Part model, mm, in its own coordinate system. A direction names the side the tool comes from. Round coordinates to 2 decimals unless told otherwise and drop trailing zeros. Loops run counter-clockwise (first coordinate to the right, second up) from the corner with the lowest first, then second, coordinate; pieces in that order, holes last. Notation, with made-up numbers: (-2, 28) - (10, 28) arc R31 ccw to (10, 59) - close; hole circle Ø9 at (8, 44). An arc over 180 degrees is marked (long way). Put each result on its own line as item: value.
from build123d import *

# Parameters (mm, degrees)
RESSALTO_EXTRUS_O1_DEPTH                     = 200
CORTE_EXTRUS_O3_REACH                        = 224.463
ESBO_O4_R                                    = 1.825
CORTE_EXTRUS_O5_REACH                        = 224.463
ESBO_O6_R                                    = 6.0125
BROCA_DE_ROSQUEAR_PARA_TARRAXA_DE_M3X0_5_D   = 2.5
ESBO_O15_W                                   = 12
ESBO_O15_H                                   = 2.152025528
CORTE_EXTRUS_O7_DEPTH                        = 16.7
CORTE_EXTRUS_O8_REACH                        = 224.463
ESBO_O5_R                                    = 6.0125
BROCA_DE_ROSQUEAR_PARA_TARRAXA_DE_M3_2_D     = 2.5
BROCA_DE_ROSQUEAR_PARA_TARRAXA_DE_M3_2_DEPTH = 2
BROCA_DE_ROSQUEAR_PARA_TARRAXA_DE_M3_3_D     = 2.5
BROCA_DE_ROSQUEAR_PARA_TARRAXA_DE_M3_3_DEPTH = 2
BROCA_DE_ROSQUEAR_PARA_TARRAXA_DE_M3_4_D     = 2.5
BROCA_DE_ROSQUEAR_PARA_TARRAXA_DE_M3_4_DEPTH = 2
BROCA_DE_ROSQUEAR_PARA_TARRAXA_DE_M3_5_D     = 2.5
BROCA_DE_ROSQUEAR_PARA_TARRAXA_DE_M3_5_DEPTH = 2


with BuildPart() as part:
    # Esboço1 → Ressalto-extrusão1 (new body)
    with BuildSketch(Plane.XY):
        Polygon((-54.740307174, -0.6), (-54.740307174, 63.2), (-71.440307174, 63.2), (-71.440307174, 65.2), (-54.740307174, 65.2), (-54.740307174, 71.2), (-71.440307174, 71.2), (-71.440307174, 73.2), (-54.740307174, 73.2), (-54.740307174, 79.2), (-73.740307174, 79.2), (-73.740307174, 83), (-71.740307174, 83), (-71.740307174, 81.2), (-59.940307174, 81.2), (-59.940307174, 91.6), (-71.740307174, 91.6), (-71.740307174, 89.8), (-73.740307174, 89.8), (-73.740307174, 93.6), (-54.940307174, 93.6), (-54.940307174, 91.6), (-56.940307174, 91.6), (-56.940307174, 83.4), (-44.540307174, 83.4), (-44.540307174, 91.6), (-46.540307174, 91.6), (-46.540307174, 93.6), (-27.740307174, 93.6), (-27.740307174, 89.8), (-29.740307174, 89.8), (-29.740307174, 91.6), (-41.540307174, 91.6), (-41.540307174, 81.2), (-29.740307174, 81.2), (-29.740307174, 83), (-27.740307174, 83), (-27.740307174, 79.2), (-46.740307174, 79.2), (-46.740307174, 71.9), (-30.040307174, 71.9), (-30.040307174, 69.9), (-46.740307174, 69.9), (-46.740307174, 62.6), (-30.040307174, 62.6), (-30.040307174, 60.6), (-46.740307174, 60.6), (-46.740307174, 53.3), (-30.040307174, 53.3), (-30.040307174, 51.3), (-46.740307174, 51.3), (-46.740307174, 11.3), (-30.040307174, 11.3), (-30.040307174, 9.3), (-46.740307174, 9.3), (-46.740307174, 2), (-30.040307174, 2), (-30.040307174, 0), (-46.740307174, 0), (-46.740307174, -7.3), (-30.040307174, -7.3), (-30.040307174, -9.3), (-46.740307174, -9.3), (-46.740307174, -16.6), (-27.740307174, -16.6), (-27.740307174, -20.4), (-29.740307174, -20.4), (-29.740307174, -18.6), (-41.540307174, -18.6), (-41.540307174, -29), (-29.740307174, -29), (-29.740307174, -27.2), (-27.740307174, -27.2), (-27.740307174, -31), (-46.540307174, -31), (-46.540307174, -29), (-44.540307174, -29), (-44.540307174, -20.8), (-56.940307174, -20.8), (-56.940307174, -29), (-54.940307174, -29), (-54.940307174, -31), (-73.740307174, -31), (-73.740307174, -27.2), (-71.740307174, -27.2), (-71.740307174, -29), (-59.940307174, -29), (-59.940307174, -18.6), (-71.740307174, -18.6), (-71.740307174, -20.4), (-73.740307174, -20.4), (-73.740307174, -16.6), (-54.740307174, -16.6), (-54.740307174, -10.6), (-71.440307174, -10.6), (-71.440307174, -8.6), (-54.740307174, -8.6), (-54.740307174, -2.6), (-71.440307174, -2.6), (-71.440307174, -0.6), align=None)
    extrude(amount=RESSALTO_EXTRUS_O1_DEPTH)

    # Esboço4 → Corte-extrusão3 (cut, up to next)
    with BuildSketch(Plane.ZY.offset(54.740307174), mode=Mode.PRIVATE) as corte_extrus_o3_sk1:
        with Locations(Location((104, 50.1, 0), (0, 0, 270))):
            Circle(ESBO_O4_R)
    corte_extrus_o3_tool1 = extrude(corte_extrus_o3_sk1.sketch, amount=-CORTE_EXTRUS_O3_REACH, mode=Mode.PRIVATE) & part.part
    add(corte_extrus_o3_tool1.solids().sort_by_distance((-54.740307, 50.1, 104))[0], mode=Mode.SUBTRACT)

    # Esboço6 → Corte-extrusão5 (cut, up to next)
    with BuildSketch(Plane.ZY.offset(54.740307174), mode=Mode.PRIVATE) as corte_extrus_o5_sk1:
        with Locations(Location((104, 12.5, 0), (0, 0, 270))):
            Circle(ESBO_O6_R)
    corte_extrus_o5_tool1 = extrude(corte_extrus_o5_sk1.sketch, amount=-CORTE_EXTRUS_O5_REACH, mode=Mode.PRIVATE) & part.part
    add(corte_extrus_o5_tool1.solids().sort_by_distance((-54.740307, 12.5, 104))[0], mode=Mode.SUBTRACT)

    # Broca de rosquear para tarraxa de M3x0.5 (through all)
    with Locations(Plane.ZY.offset(54.740307174)):
        with Locations((6, 5.9), (6, 58.2)):
            Hole(BROCA_DE_ROSQUEAR_PARA_TARRAXA_DE_M3X0_5_D / 2)

    # Esboço15 → Corte-extrusão7 (cut)
    with BuildSketch(Plane(origin=(-30.040307174, 0, 0), x_dir=(0, 0, -1), z_dir=(1, 0, 0))):
        with Locations((-104.566575702, 52.223987236)):
            Rectangle(ESBO_O15_W, ESBO_O15_H)
    extrude(amount=-CORTE_EXTRUS_O7_DEPTH, mode=Mode.SUBTRACT)

    # Esboço5 → Corte-extrusão8 (cut, up to next)
    with BuildSketch(Plane.ZY.offset(54.740307174), mode=Mode.PRIVATE) as corte_extrus_o8_sk1:
        with Locations(Location((130, 50.1, 0), (0, 0, 270))):
            Circle(ESBO_O5_R)
    corte_extrus_o8_tool1 = extrude(corte_extrus_o8_sk1.sketch, amount=-CORTE_EXTRUS_O8_REACH, mode=Mode.PRIVATE) & part.part
    add(corte_extrus_o8_tool1.solids().sort_by_distance((-54.740307, 50.1, 130))[0], mode=Mode.SUBTRACT)

    # Broca de rosquear para tarraxa de M3 2
    with Locations(Plane.XZ.offset(31)):
        with Locations((-64.286083069, 189.76), (-37.140307173, 189.76)):
            Hole(BROCA_DE_ROSQUEAR_PARA_TARRAXA_DE_M3_2_D / 2, depth=BROCA_DE_ROSQUEAR_PARA_TARRAXA_DE_M3_2_DEPTH)

    # Broca de rosquear para tarraxa de M3 3
    with Locations(Plane(origin=(0, 93.6, 0), x_dir=(-1, 0, 0), z_dir=(0, 1, 0))):
        with Locations((37.140307173, 189.76), (64.340307173, 189.76)):
            Hole(BROCA_DE_ROSQUEAR_PARA_TARRAXA_DE_M3_3_D / 2, depth=BROCA_DE_ROSQUEAR_PARA_TARRAXA_DE_M3_3_DEPTH)

    # Broca de rosquear para tarraxa de M3 4
    with Locations(Plane.XZ.offset(31)):
        with Locations((-64.340307174, 18.36), (-64.340307174, 6.36)):
            Hole(BROCA_DE_ROSQUEAR_PARA_TARRAXA_DE_M3_4_D / 2, depth=BROCA_DE_ROSQUEAR_PARA_TARRAXA_DE_M3_4_DEPTH)

    # Broca de rosquear para tarraxa de M3 5
    with Locations(Plane(origin=(0, 93.6, 0), x_dir=(-1, 0, 0), z_dir=(0, 1, 0))):
        with Locations((64.340307174, 18.36), (64.340307174, 6.36)):
            Hole(BROCA_DE_ROSQUEAR_PARA_TARRAXA_DE_M3_5_D / 2, depth=BROCA_DE_ROSQUEAR_PARA_TARRAXA_DE_M3_5_DEPTH)


solid = part.part
1. Two-plate mould, pull along Z, no slides. Class faces 1 (the flat face through (-36, 81.2, 99)), 2 (the cylindrical face through (-48.05, 51.4, 124.13)), 3 (the flat face through (-54, 32, 0)): pulls with the +Z half, pulls with the -Z half, needs draft (parallel to the pull), parting line crosses it, or undercut.
A:
face 1: needs draft
face 2: undercut
face 3: pulls with the -Z half
2. Band-saw the part on B-B (y = 33.5). List the corners of the cut face in (x, z).
A:
outline: (-54.74, 0) - (-46.74, 0) - (-46.74, 200) - (-54.74, 200) - close
3. Pin check, flat tips, straight feed: P1, Ø4, axis at y = 27.5, z = 41, coming from the +X side; P2, Ø3, axis at x = -49.5, z = 73, coming from the +Y side; P3, Ø1.6, axis at y = 52.5, z = 116.5, coming from the +X side. Stop position of each tip, or through.
A:
P1: stops at x = -46.74
P2: stops at y = 83.4
P3: stops at x = -30.04
4. Probe line 1 along Z through (x, y) = (-50.75, 50.1) (1 decimal); line 2 along X through (y, z) = (84.5, 96.5); line 3 along X through (y, z) = (-30.25, 189.76). List the from-to ranges inside material, lowest first. Write a range as [from, to].
A:
line 1: z = [0, 102.2], [105.8, 124], [136, 200]
line 2: x = [-59.94, -56.94], [-44.54, -41.54]
line 3: x = [-73.74, -65.54], [-63.04, -54.94], [-46.54, -38.39], [-35.89, -27.74]
5. Tool access for faces 4 (the flat face through (-38, 60.6, 99)), 5 (the flat face through (-63, -8.6, 99)), 6 (the flat face through (-66, -29, 99)), 7 (the flat face through (-73.74, 92, 99)): list every direction of +Z, -Z, +X, -X, +Y, -Y with a clear straight run to the whole face (end or side of a thin tool).
A:
face 4: +Z, -Z, +X
face 5: +Z, -Z, -X
face 6: +Z, -Z
face 7: +Z, -Z, -X, +Y, -Y
6. Band-saw the part on A-A (x = -51.5). Give the number of separate pieces and of enclosed holes in the cut face, plus the area to 3 significant figures.
A:
separate pieces: 1
enclosed holes: 5
area: 20,600 mm²
